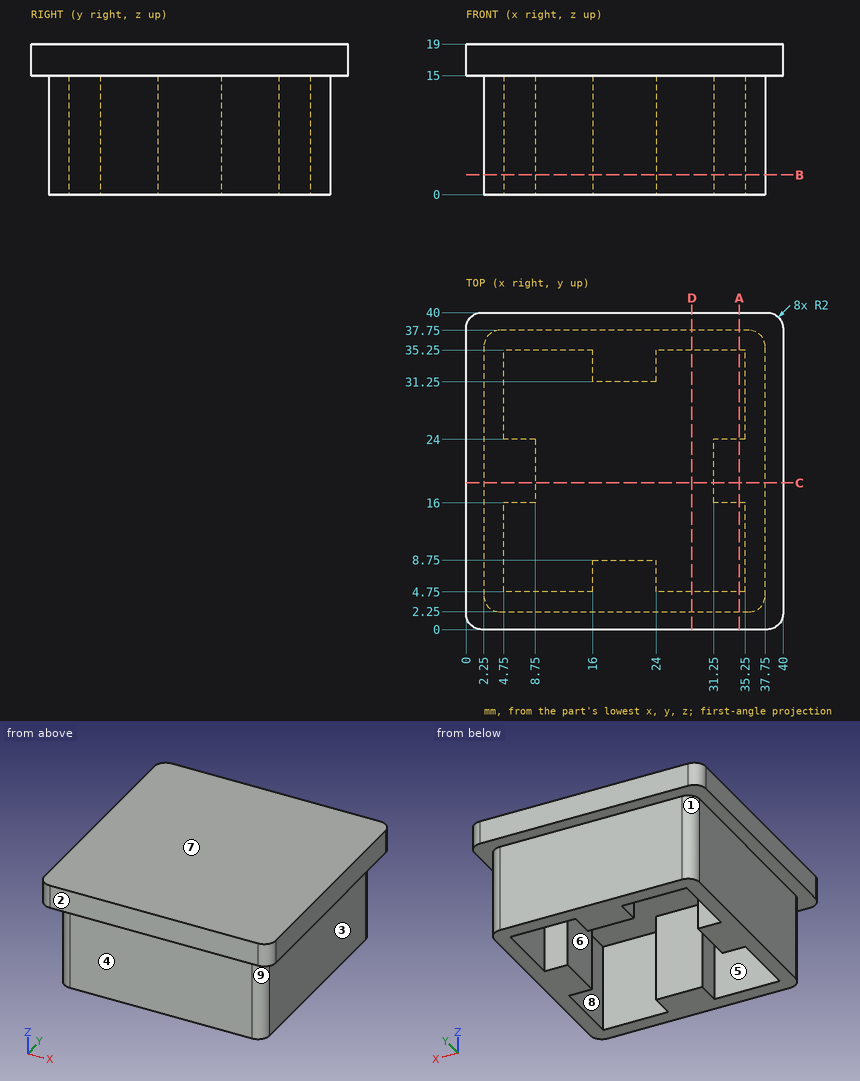
Source: three-view drawing plus pictorial views. Frame: mm from the lowest corner of the part. A direction names the side the tool comes from. Coordinates: 2 decimals unless noted, no trailing zeros. Loops run counter-clockwise (first coordinate to the right, second up) from the corner with the lowest first, then second, coordinate; pieces in that order, holes last. Notation, with made-up numbers: (77.5, 3.5) -> (85.5, 3.5) arc R36 ccw to (85.5, 38.5) -> close; hole circle Ø4 at (-27, -33.5). An arc over 180 degrees is marked (long way). Write each question's results on one line, items separated by ' | '. Start each with the question number.
Q1. Section D-D, the plane x = 28.5. Return the cut outline in (y, z), plus the area to 3 significant figures.
Q2. Reachability of the marked faces 1, 2, 3, 4 and 5 from +Z, -Z, +X, -X, +Y, -Y: full face, straight path, thin tool, end or side. Return the list, or none.
Q3. Section C-C, the plane y = 18.5. Return the cut outline in (x, z), plus the area to 3 significant figures.
Q4. Pin query (flat end, axial travel): pin 1 (1.5 mm diameter, centred on y = 33.5, z = 13, fed in from -X); pin 2 (2 mm diameter, centred on x = 7.5, z = 9, fed in from +Y); pin 3 (2.5 mm diameter, centred on x = 19.5, z = 10, fed in from -Y). Return the tip coordinate at first contact, or that it passes through.
Q5. Ray query, line 1 (X direction, y = 5, z = 7); line 2 (Y direction, x = 12.5, z = 1); line 3 (X direction, y = 22, z = 13.75). Return the intervals inside material, ascending. Write a range as from..to.
Q6. Section B-B, the plane z = 2.5. Return the cut outline in (x, y), plus the area to 3 significant figures.
Q7. Pull-direction query (Y, two-part tool) for the marked faces 6, 7, 8 and 9; classes: released by +Y, released by -Y, zero draft, split by the parting line, or undercut.
Q8. Section A-A, the plane x = 34.5. Return the cut outline in (y, z), plus the area to 3 significant figures.
Found:
1) outline: (0, 15) -> (2.25, 15) -> (2.25, 0) -> (4.75, 0) -> (4.75, 15) -> (35.25, 15) -> (35.25, 0) -> (37.75, 0) -> (37.75, 15) -> (40, 15) -> (40, 19) -> (0, 19) -> close | area: 235 mm2
2) face 1: -Z, -X, +Y | face 2: +Z, -Z, +X, -X, -Y | face 3: -Z, +X, +Y, -Y | face 4: -Z, +X, -X, -Y | face 5: -Z
3) outline: (0, 15) -> (2.25, 15) -> (2.25, 0) -> (8.75, 0) -> (8.75, 15) -> (31.25, 15) -> (31.25, 0) -> (37.75, 0) -> (37.75, 15) -> (40, 15) -> (40, 19) -> (0, 19) -> close | area: 355 mm2
4) pin 1: x = 2.25 | pin 2: y = 37.75 | pin 3: y = 2.25
5) line 1: 2.25..4.75, 16..24, 35.25..37.75 | line 2: 2.25..4.75, 35.25..37.75 | line 3: 2.25..8.75, 31.25..37.75
6) outline: (2.25, 4.25) arc R2 ccw to (4.25, 2.25) -> (35.75, 2.25) arc R2 ccw to (37.75, 4.25) -> (37.75, 35.75) arc R2 ccw to (35.75, 37.75) -> (4.25, 37.75) arc R2 ccw to (2.25, 35.75) -> close; hole (4.75, 4.75) -> (16, 4.75) -> (16, 8.75) -> (24, 8.75) -> (24, 4.75) -> (35.25, 4.75) -> (35.25, 16) -> (31.25, 16) -> (31.25, 24) -> (35.25, 24) -> (35.25, 35.25) -> (24, 35.25) -> (24, 31.25) -> (16, 31.25) -> (16, 35.25) -> (4.75, 35.25) -> (4.75, 24) -> (8.75, 24) -> (8.75, 16) -> (4.75, 16) -> close | area: 455 mm2
7) face 6: undercut | face 7: zero draft | face 8: undercut | face 9: released by -Y
8) outline: (0, 15) -> (2.25, 15) -> (2.25, 0) -> (4.75, 0) -> (4.75, 15) -> (16, 15) -> (16, 0) -> (24, 0) -> (24, 15) -> (35.25, 15) -> (35.25, 0) -> (37.75, 0) -> (37.75, 15) -> (40, 15) -> (40, 19) -> (0, 19) -> close | area: 355 mm2
